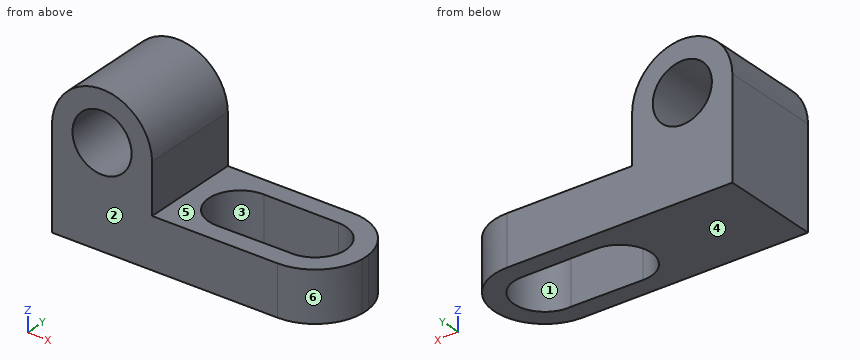
from build123d import *

# Parameters (mm, degrees)
F1_DEPTH  = 25.4
F2_R      = 7.491958629
F3_DEPTH  = 25.401
F5_DEPTH  = 25.401
F6_R      = 7.8989022762
F6_R_2    = 7.7951690208
F7_DEPTH  = 12.701
F9_DEPTH  = 12.701
F11_DEPTH = 12.701


with BuildPart() as f1:
    # F0 (on Front) → F1 (new body)
    with BuildSketch(Plane.XZ):
        Polygon((-53.5450525341, 38.1), (-78.9450525341, 38.1), (-78.9450525341, 0), (-9.0950525341, 0), (-9.0950525341, 12.7), (-53.5450525341, 12.7), align=None)
    extrude(amount=F1_DEPTH)

    # F2 (on face) → F3 (cut, through all)
    with BuildSketch(Plane.XZ.offset(25.4)):
        with Locations((-66.2450525341, 25.4)):
            Circle(F2_R)
    extrude(amount=-F3_DEPTH, mode=Mode.SUBTRACT)

    # F4 (on face) → F5 (cut, through all)
    with BuildSketch(Plane.XZ.offset(25.4)):
        with BuildLine():
            ThreePointArc((-78.9450525341, 25.4), (-66.2450525341, 37.895691554), (-53.5450525341, 25.4))
            Line((-53.5450525341, 25.4), (-53.5450525341, 38.1))
            Line((-53.5450525341, 38.1), (-78.9450525341, 38.1))
            Line((-78.9450525341, 38.1), (-78.9450525341, 25.4))
        make_face()
    extrude(amount=-F5_DEPTH, mode=Mode.SUBTRACT)

    # F6 (on face) → F7 (cut, through all)
    with BuildSketch(Plane.XY.offset(12.7)):
        with Locations((-40.8450525341, -12.7)):
            Circle(F6_R)
        with Locations((-21.7950525341, -12.7)):
            Circle(F6_R_2)
    extrude(amount=-F7_DEPTH, mode=Mode.SUBTRACT)

    # F8 (on face) → F9 (cut, through all)
    with BuildSketch(Plane.XY.offset(12.7)):
        with BuildLine():
            ThreePointArc((-32.9461502579, -12.7), (-35.204801221, -18.2299387243), (-40.6890545818, -20.5973616992))
            Line((-40.6890545818, -20.5973616992), (-22.5810122533, -20.4554450151))
            ThreePointArc((-22.5810122533, -20.4554450151), (-29.5791895595, -12.2854269284), (-21.7528127547, -4.9049454227))
            Line((-21.7528127547, -4.9049454227), (-40.7127795229, -4.8022053066))
            ThreePointArc((-40.7127795229, -4.8022053066), (-35.2131137579, -7.1615956459), (-32.9461502579, -12.7))
        make_face()
    extrude(amount=-F9_DEPTH, mode=Mode.SUBTRACT)

    # F10 (on face) → F11 (cut, through all)
    with BuildSketch(Plane.XY.offset(12.7)):
        with BuildLine():
            ThreePointArc((-21.7528127547, 0), (-13.1462388454, -3.3610018984), (-9.0950525341, -11.6650573949))
            Line((-9.0950525341, -11.6650573949), (-9.0950525341, 0))
            Line((-9.0950525341, 0), (-21.7528127547, 0))
        make_face()
        with BuildLine():
            ThreePointArc((-9.0950525341, -13.7349426051), (-13.1462388454, -22.0389981016), (-21.7528127547, -25.4))
            Line((-21.7528127547, -25.4), (-9.0950525341, -25.4))
            Line((-9.0950525341, -25.4), (-9.0950525341, -13.7349426051))
        make_face()
    extrude(amount=-F11_DEPTH, mode=Mode.SUBTRACT)


solid = f1.part
Check sheet for the modelled part. Datum: model origin and axes. Units: mm. Face numbers are marked on the shaded views. A direction names the side the tool comes from. Round coordinates to 2 decimals unless told otherwise and drop trailing zeros. Loops run counter-clockwise (first coordinate to the right, second up) from the corner with the lowest first, then second, coordinate; pieces in that order, holes last. Notation, with made-up numbers: (18, 41.25) -> (49, 41.25) arc R19 ccw to (49, 76.25) -> close; hole circle Ø6 at (50.5, -34). An arc over 180 degrees is marked (long way). Put each result on its own line as item: value. Start each with the question number.
1. Section check B-B (z = 29). Enter the section's corners in (x, y).
2. Scan lines: probe 1 along Z at (x, y) = (-20, -23); probe 2 along Z at (x, y) = (-70.5, -20.25); probe 3 along Y at (x, z) = (-48, 2). Record each from-to range of solid material in increasing order.
3. Section check C-C (x = -69). Enter the section's corners in (y, z).
4. Draft check along Y on the marked faces 1, 2, 3 and 4. Enter one of: +Y half, -Y half, draft (parallel to the pull), parting line (faces both ways), or undercut.
5. Gauge pin test, flat ends, axial feed: pin 1 (2 mm diameter, centred on y = -20, z = 29, fed in from -X); pin 2 (1 mm diameter, centred on y = -10.5, z = 22, fed in from +X); pin 3 (3 mm diameter, centred on x = -68.5, y = -18.5, fed in from +Z). Record the tip position at first contact, or that the pin passes through.
6. Access from +Z, -Z, +X, -X, +Y, -Y to the whole of each face (thin tool, end or side, straight path). Record for the marked faces 5 and 6.
Findings:
1. outline: (-78.36, -25.4) -> (-72.82, -25.4) -> (-72.82, 0) -> (-78.36, 0) -> close; (-59.67, -25.4) -> (-54.13, -25.4) -> (-54.13, 0) -> (-59.67, 0) -> close
2. probe 1: z = 0 to 12.7
2. probe 2: z = 0 to 19.23, 31.57 to 37.16
2. probe 3: y = -25.4 to -16.05, -9.35 to 0
3. outline: (-25.4, 0) -> (0, 0) -> (0, 18.43) -> (-25.4, 18.43) -> close; (-25.4, 32.37) -> (0, 32.37) -> (0, 37.59) -> (-25.4, 37.59) -> close
4. face 1: undercut
4. face 2: -Y half
4. face 3: undercut
4. face 4: draft
5. pin 1: stops at x = -78.63
5. pin 2: stops at x = -53.55
5. pin 3: stops at z = 37.87
6. face 5: +Z, +X, +Y, -Y
6. face 6: +Z, -Z, +X, -Y
